```python
from build123d import *

# Parameters (mm, degrees)
F0_R     = 63.918721
F0_R_2   = 56.918721
F1_DEPTH = 25.4
F2_R     = 11.15
F3_DEPTH = 76.2
F4_R     = 11.1506
F5_DEPTH = 76.2
F6_R     = 11.1506
F7_DEPTH = 76.2
F8_R     = 11.1506
F9_DEPTH = 76.2


with BuildPart() as f1:
    # F0 (on Top) → F1 (new body)
    with BuildSketch(Plane.XY):
        Circle(F0_R)
        Circle(F0_R_2, mode=Mode.SUBTRACT)
    extrude(amount=F1_DEPTH)

    # F2 (on Front) → F3 (cut)
    with BuildSketch(Plane.XZ):
        with Locations((0, 12.7)):
            Circle(F2_R)
    extrude(amount=F3_DEPTH, mode=Mode.SUBTRACT)

    # F4 (on Front) → F5 (cut)
    with BuildSketch(Plane.XZ):
        with Locations((0, 12.7)):
            Circle(F4_R)
    extrude(amount=-F5_DEPTH, mode=Mode.SUBTRACT)

    # F6 (on Right) → F7 (cut)
    with BuildSketch(Plane.YZ):
        with Locations((0, 12.7)):
            Circle(F6_R)
    extrude(amount=-F7_DEPTH, mode=Mode.SUBTRACT)

    # F8 (on Right) → F9 (cut)
    with BuildSketch(Plane.YZ):
        with Locations((0, 12.7)):
            Circle(F8_R)
    extrude(amount=F9_DEPTH, mode=Mode.SUBTRACT)


solid = f1.part
```
CAD build for the part. Positions are in the model's coordinates, mm. Give positions to 0.01 mm unless a question says otherwise; leave off trailing zeros. Write each loop counter-clockwise with the first axis right and the second up, starting at its lowest first coordinate (ties: lowest second). Pieces come first, ordered by that corner, then holes. Notation, with made-up numbers: M 35.25,60 L 91.25,60 A11 cw 91.25,69 Z; hole C -1.5,-3 d7. An arc over 180 degrees is marked long. Return JSON: item names as keys, results as strings. Group by question number.
(1) Band-saw the part on D-D (x = -45.5). Give the cut face in (y, z).
(2) Band-saw the part on C-C (z = 15). Give the cut face in (x, y).
(3) Drill centre lines: L1, parallel to Z at x = 59, y = 0; L2, parallel to X at y = 47.5, z = 6.75. Where is each one in solid material? Low to high. Write a range as [from, to].
(4) Band-saw the part on A-A (x = 0). Give the cut face in (y, z).
(5) Band-saw the part on B-B (y = 39.5). Give the cut face in (x, z), and give its area (3 significant figures).
(6) Mould opens along Z. For faces 1 (the face through (-43, -38, 0)), 2 (the face through (-43, -38, 25.4)), 3 (the face through (10.3, 59.81, 8.43)), 4 (the face through (-59.81, 10.3, 8.43)) say: pulls with the +Z half, pulls with the -Z half, needs draft (parallel to the pull), parting line crosses it, or undercut.
(7) Flat gauge pins, fed straight in: pin 1 Ø12 at (x, z) = (47, 4) entering from +Y; pin 2 Ø8 at (y, z) = (-26.5, 12) entering from +X; pin 3 Ø8 at (x, z) = (20.5, 10) entering from +Y; pin 4 Ø13.5 at (x, z) = (0, 12.7) entering from +Y. Where does each tip first touch, or does it go through?
Entries:
{
 "1": {"outline": "M -44.89,0 L -34.2,0 L -34.2,25.4 L -44.89,25.4 Z; M 34.2,0 L 44.89,0 L 44.89,25.4 L 34.2,25.4 Z"},
 "2": {"outline": "M -62.98,-10.91 A63.92 ccw -10.91,-62.98 L -10.91,-55.86 A56.92 cw -55.86,-10.91 Z; M -62.98,10.91 L -55.86,10.91 A56.92 cw -10.91,55.86 L -10.91,62.98 A63.92 ccw Z; M 10.91,-62.98 A63.92 ccw 62.98,-10.91 L 55.86,-10.91 A56.92 cw 10.91,-55.86 Z; M 10.91,55.86 A56.92 cw 55.86,10.91 L 62.98,10.91 A63.92 ccw 10.91,62.98 Z"},
 "3": {"L1": "z = [0, 1.55], [23.85, 25.4]", "L2": "x = [-42.77, -31.36], [31.36, 42.77]"},
 "4": {"outline": "M -63.92,0 L -56.92,0 L -56.92,1.55 L -63.92,1.55 Z; M -63.92,23.85 L -56.92,23.85 L -56.92,25.4 L -63.92,25.4 Z; M 56.92,0 L 63.92,0 L 63.92,1.55 L 56.92,1.55 Z; M 56.92,23.85 L 63.92,23.85 L 63.92,25.4 L 56.92,25.4 Z"},
 "5": {"outline": "M -50.25,0 L -40.98,0 L -40.98,25.4 L -50.25,25.4 Z; M 40.98,0 L 50.25,0 L 50.25,25.4 L 40.98,25.4 Z", "area": "471 mm^2"},
 "6": {"face 1": "pulls with the -Z half", "face 2": "pulls with the +Z half", "face 3": "undercut", "face 4": "undercut"},
 "7": {"pin 1": "stops at y = 49.04", "pin 2": "stops at x = 59.83", "pin 3": "stops at y = 61.75", "pin 4": "passes through"}
}
